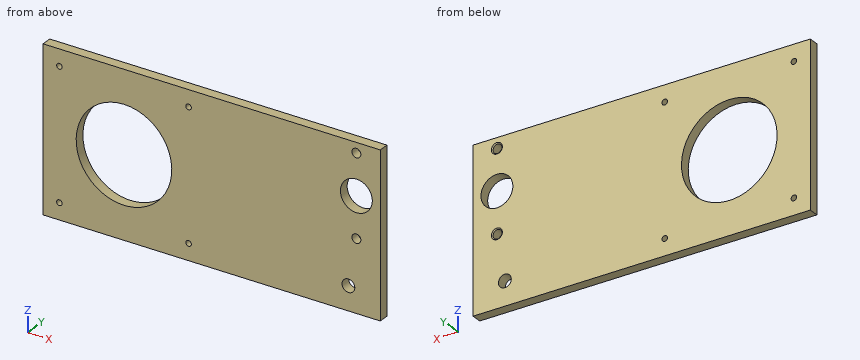
```python
from build123d import *

# Parameters (mm, degrees)
SKETCH1_W                        = 211.6
SKETCH1_H                        = 101.6
SKETCH1_R                        = 30
SKETCH1_R_2                      = 4.025
SKETCH1_R_3                      = 10
BOSS_EXTRUDE1_DEPTH              = 6.35
F_8_32_TAPPED_HOLE1_D            = 3.4544
F_10_CLEARANCE_HOLE1_D           = 5.6134
F_10_CLEARANCE_HOLE1_CSINK_D     = 6.8834
F_10_CLEARANCE_HOLE1_CSINK_ANGLE = 90


with BuildPart() as part:
    # Sketch1 → Boss-Extrude1 (new body)
    with BuildSketch(Plane(origin=(0, 0, 0), x_dir=(1, 0, 0), z_dir=(0, 1, 0))):
        with Locations((55, 0)):
            Rectangle(SKETCH1_W, SKETCH1_H)
        with Locations(Location((0, 0, 0), (0, 0, 270))):
            Circle(SKETCH1_R, mode=Mode.SUBTRACT)
        with Locations(Location((140.8, 35.8, 0), (0, 0, 270))):
            Circle(SKETCH1_R_2, mode=Mode.SUBTRACT)
        with Locations(Location((145.8, -19.05, 0), (0, 0, 270))):
            Circle(SKETCH1_R_3, mode=Mode.SUBTRACT)
    extrude(amount=BOSS_EXTRUDE1_DEPTH)

    # #8-32 Tapped Hole1 (through all)
    with Locations(Plane(origin=(0, 6.35, 0), x_dir=(1, 0, 0), z_dir=(0, 1, 0))):
        with Locations((-40.513, 40.513), (40.513, 40.513), (40.513, -40.513), (-40.513, -40.513)):
            Hole(F_8_32_TAPPED_HOLE1_D / 2)

    # #10 Clearance Hole1 (through all)
    with Locations(Plane(origin=(0, 6.35, 0), x_dir=(1, 0, 0), z_dir=(0, 1, 0))):
        with Locations((145.8, 6.35), (145.8, -44.45)):
            CounterSinkHole(F_10_CLEARANCE_HOLE1_D / 2, F_10_CLEARANCE_HOLE1_CSINK_D / 2, counter_sink_angle=F_10_CLEARANCE_HOLE1_CSINK_ANGLE)


solid = part.part
```
The listing builds one solid part. Answer for the finished solid, in the listing's coordinates (mm). Give positions to 0.01 mm unless a question says otherwise; leave off trailing zeros. Order: outer loops, then holes, each group sorted by start corner. A loop starts at its lowest first (then second) coordinate and runs counter-clockwise, first axis right, second up. Notation, with made-up numbers: (-34, 59) - (4, 59) arc R14 cw to (4, 74) - close; hole circle Ø8 at (23, 31.25). An arc over 180 degrees is marked (long way). Use one line per item in the form item = value. Start each with the question number.
(1) A cutting plane is placed at C-C, the plane z = -6.35. Write down the section's boundary in (x, y) (3 decimals).
(2) A cutting plane is placed at D-D, the plane y = 4.75. State how many separate pieces and enclosed holes the cut face has, then the cut area to 3 significant figures.
(3) A flat-ended cylindrical pin translates along its axis: pin 1 Ø4.5 at (x, z) = (145.8, 44.45) entering from +Y. Find the tip coordinate at first contact, or state that the pin passes through.
(4) A cutting plane is placed at B-B, the plane x = -5.5. Write down the section's boundary in (y, z).
(5) Consider line 1 (Z direction, x = 139.5, y = 1.5); line 2 (X direction, y = 5.25, z = -35.8) (3 decimals); line 3 (X direction, y = 3.25, z = 44.45). Determine where each line is inside the solid, lowest interval first. Write a range as from..to.
(6) A cutting plane is placed at A-A, the plane z = 44.45. Write down the section's boundary in (x, y) (3 decimals).
Ans:
q1.outline = (-50.8, 0) - (-29.32, 0) - (-29.32, 6.35) - (-50.8, 6.35) - close; (29.32, 0) - (142.993, 0) - (142.993, 5.715) - (142.358, 6.35) - (29.32, 6.35) - close; (148.607, 0) - (160.8, 0) - (160.8, 6.35) - (149.242, 6.35) - (148.607, 5.715) - close
q2.separate_pieces = 1
q2.enclosed_holes = 9
q2.area = 18,200 mm^2
q3.pin_1 = through
q4.outline = (0, -50.8) - (6.35, -50.8) - (6.35, -29.49) - (0, -29.49) - close; (0, 29.49) - (6.35, 29.49) - (6.35, 50.8) - (0, 50.8) - close
q5.line_1 = -50.8..-39.61, -31.99..11.28, 26.82..50.8
q5.line_2 = -50.8..136.775, 144.825..160.8
q5.line_3 = -50.8..142.99, 148.61..160.8
q6.outline = (-50.8, 0) - (142.993, 0) - (142.993, 5.715) - (142.358, 6.35) - (-50.8, 6.35) - close; (148.607, 0) - (160.8, 0) - (160.8, 6.35) - (149.242, 6.35) - (148.607, 5.715) - close
